```python
from build123d import *

# Parameters (mm, degrees)
ESQUISSE4_W                                      = 275
ESQUISSE4_H                                      = 157
BOSS_EXTRU_2_DEPTH                               = 4
FRAISAGE_POUR_VIS_T_TE_FRAIS_E_M42_AT_COUNT      = 2
FRAISAGE_POUR_VIS_T_TE_FRAIS_E_M42_AT_PITCH      = 235.512207752
FRAISAGE_POUR_VIS_T_TE_FRAIS_E_M42_2_COUNT       = 2
FRAISAGE_POUR_VIS_T_TE_FRAIS_E_M42_2_PITCH       = 229
FRAISAGE_POUR_VIS_T_TE_FRAIS_E_M42_3_COUNT       = 2
FRAISAGE_POUR_VIS_T_TE_FRAIS_E_M42_3_PITCH       = 55
CHAMBRAGE_POUR_VIS_T_TE_RONDE_6_PANS_D           = 6.6
CHAMBRAGE_POUR_VIS_T_TE_RONDE_6_PANS_CBORE_D     = 11.5
CHAMBRAGE_POUR_VIS_T_TE_RONDE_6_PANS_CBORE_DEPTH = 2
CONG_1_R                                         = 9
CONG_2_R                                         = 2


with BuildPart() as part:
    # Esquisse4 → Boss.-Extru.2 (new body)
    with BuildSketch(Plane.XY):
        Rectangle(ESQUISSE4_W, ESQUISSE4_H)
    extrude(amount=BOSS_EXTRU_2_DEPTH)

    # Esquisse6 → Fraisage pour vis à tête fraisée M42 (revolve, cut)
    with BuildSketch(Plane(origin=(-114.5, -21, 0), x_dir=(0, 1, 0), z_dir=(1, 0, 0))):
        Polygon((0, 0), (0, 4), (2.25, 4), (2.25, 2.45), (4.7, 0), align=None)
    fraisage_pour_vis_t_te_frais_e_m42 = revolve(axis=Axis((-114.5, -21, -6.35), (0, 0, 1)), mode=Mode.SUBTRACT)

    # Fraisage pour vis à tête fraisée M42 at: Fraisage pour vis à tête fraisée M42 ×2
    with Locations(*[Vector(0.972348747, 0.233533542, 0) * (i * FRAISAGE_POUR_VIS_T_TE_FRAIS_E_M42_AT_PITCH) for i in range(1, FRAISAGE_POUR_VIS_T_TE_FRAIS_E_M42_AT_COUNT)]):
        add(fraisage_pour_vis_t_te_frais_e_m42, mode=Mode.SUBTRACT)

    # Fraisage pour vis _ t_te frais_e M42 2: Fraisage pour vis à tête fraisée M42 ×2
    with Locations(*[(i * FRAISAGE_POUR_VIS_T_TE_FRAIS_E_M42_2_PITCH, 0, 0) for i in range(1, FRAISAGE_POUR_VIS_T_TE_FRAIS_E_M42_2_COUNT)]):
        add(fraisage_pour_vis_t_te_frais_e_m42, mode=Mode.SUBTRACT)

    # Fraisage pour vis _ t_te frais_e M42 3: Fraisage pour vis à tête fraisée M42 ×2
    with Locations(*[(0, i * FRAISAGE_POUR_VIS_T_TE_FRAIS_E_M42_3_PITCH, 0) for i in range(1, FRAISAGE_POUR_VIS_T_TE_FRAIS_E_M42_3_COUNT)]):
        add(fraisage_pour_vis_t_te_frais_e_m42, mode=Mode.SUBTRACT)

    # Chambrage pour Vis à tête ronde à 6 pans creux M61 (through all)
    with Locations(Plane.XY.offset(4)):
        with Locations((128.5, -69.5), (-128.5, -69.5), (-128.5, 69.5), (128.5, 69.5)):
            CounterBoreHole(CHAMBRAGE_POUR_VIS_T_TE_RONDE_6_PANS_D / 2, CHAMBRAGE_POUR_VIS_T_TE_RONDE_6_PANS_CBORE_D / 2, CHAMBRAGE_POUR_VIS_T_TE_RONDE_6_PANS_CBORE_DEPTH)

    # Congé1
    cong_1_edges = [part.edges().sort_by_distance(p)[0] for p in [
        (137.5, 78.5, 2),
        (137.5, -78.5, 2),
        (-137.5, -78.5, 2),
        (-137.5, 78.5, 2),
    ]]
    fillet(cong_1_edges, radius=CONG_1_R)

    # Congé2
    cong_2_edges = [part.edges().sort_by_distance(p)[0] for p in [
        (0, 78.5, 4),
        (137.5, 0, 4),
        (-137.5, 0, 4),
        (0, -78.5, 4),
        (-134.863961031, -75.863961031, 4),
        (-134.863961031, 75.863961031, 4),
        (134.863961031, -75.863961031, 4),
        (134.863961031, 75.863961031, 4),
    ]]
    fillet(cong_2_edges, radius=CONG_2_R)


solid = part.part
```
Check sheet for the modelled part. Datum: model origin and axes. Units: mm. A direction names the side the tool comes from. Round coordinates to 2 decimals unless told otherwise and drop trailing zeros. Write item = value, one per line. Start each with the question number.
Q1. Access from +Z, -Z, +X, -X, +Y, -Y to the whole of each face (thin tool, end or side, straight path). Record for faces 1 (the face through (-126.07, 71.73, 0.99)), 2 (the face through (133.984, 71.227, 3.014)).
Q2. Release check for a two-part mould opening along X. For faces 3 (the face through (-2, 1, 4)), 4 (the face through (-134.934, -75.794, 1.014)), 5 (the face through (131, 67, 2)) record: pulls with the +X half, pulls with the -X half, needs draft (parallel to the pull), parting line crosses it, or undercut.
Q3. Depth check by flat-ended pin: P1, Ø7, axis at x = 128.5, y = -69.5, coming from the +Z side; P2, Ø6, axis at x = -114.5, y = -21, coming from the -Z side; P3, Ø5, axis at x = 114.5, y = 34, coming from the -Z side. Enter the tip coordinate at first touch or a pass-through.
Q4. Thickness scan on L1, parallel to Y at x = 128.5, z = 1.55; L2, parallel to X at y = 35, z = 2.4; L3, parallel to Y at x = -128.5, z = 3.6. Record the ranges inside material, lowest first.
Derived:
q1.face_1 = +Z, -Z
q1.face_2 = +Z
q2.face_3 = needs draft
q2.face_4 = pulls with the -X half
q2.face_5 = undercut
q3.P1 = 2
q3.P2 = 1.7
q3.P3 = 2.2
q4.L1 = -78.5 to -72.8, -66.2 to 66.2, 72.8 to 78.5
q4.L2 = -137.46 to -116.57, -112.43 to 112.43, 116.57 to 137.46
q4.L3 = -77.7 to -75.25, -63.75 to 63.75, 75.25 to 77.7
